Can you work these out from the drawing? Everything is in mm from the part's minimum corner. A direction names the side the tool comes from. Round coordinates to 2 decimals unless told otherwise and drop trailing zeros. Order: outer loops, then holes, each group sorted by start corner. A loop starts at its lowest first (then second) coordinate and runs counter-clockwise, first axis right, second up. Notation, with made-up numbers: (-16.75, -2.75) - (-0.75, -2.75) arc R24 cw to (-0.75, 7.25) - close; hole circle Ø8 at (62.25, 49). An arc over 180 degrees is marked (long way). Answer as a JSON object with one key per item and string values.
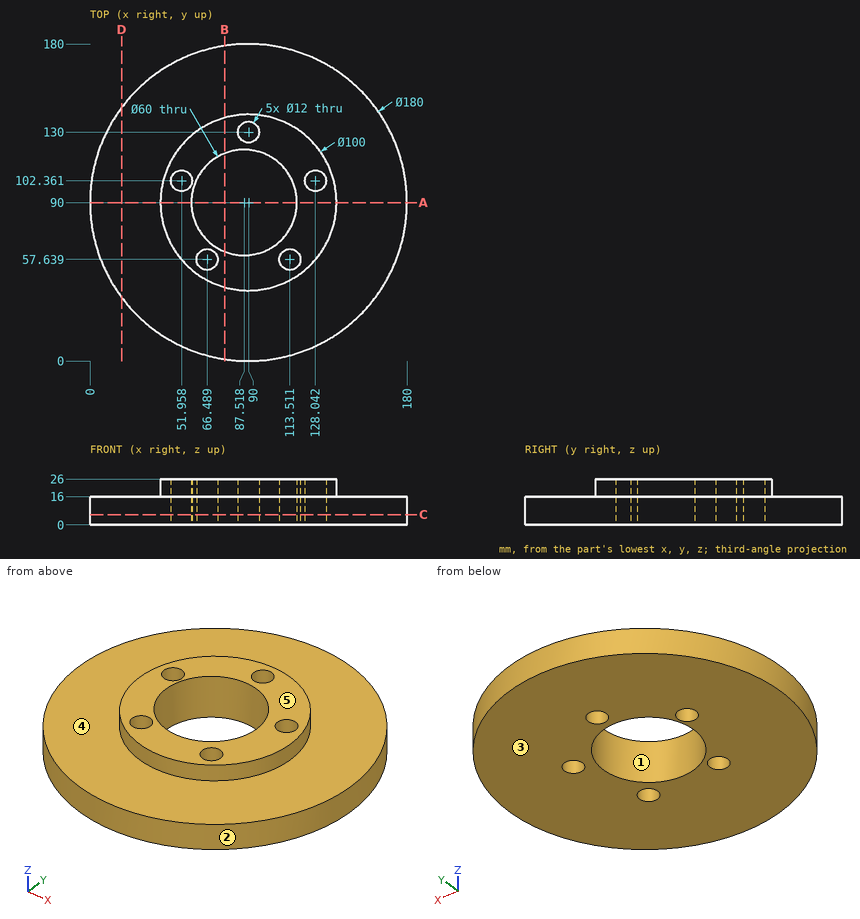
1. Imagine slicing it at C-C (z = 5.75). List the corners of the cut face in (x, y) for me, plus the area to 3 significant figures.
Responses:
{"outline": "circle Ø180 at (90, 90); hole circle Ø12 at (51.96, 102.36); hole circle Ø60 at (87.52, 90); hole circle Ø12 at (66.49, 57.64); hole circle Ø12 at (90, 130); hole circle Ø12 at (113.51, 57.64); hole circle Ø12 at (128.04, 102.36)", "area": "22,100 mm2"}
2. If I drill on L1, parallel to Y at x = 94.5, z = 12.75 (1 decimal); L2, parallel to Y at x = 114, z = 11.5 (1 decimal); L3, parallel to Z at x = 44.5, y = 50, over which ranges is the centre line in solid material (lowest first)? Write a range as [from, to].
Responses:
{"L1": "[0.1, 60.8], [119.2, 126], [134, 179.9]", "L2": "[3.3, 51.7], [63.6, 75.9], [104.1, 176.7]", "L3": "[0, 16]"}
3. Imagine slicing it at D-D (x = 18). List the corners of the cut face in (y, z) for me.
Responses:
{"outline": "(36, 0) - (144, 0) - (144, 16) - (36, 16) - close"}
4. Imagine slicing it at A-A (y = 90). List the corners of the cut face in (x, z) for me.
Responses:
{"outline": "(0, 0) - (57.52, 0) - (57.52, 26) - (40, 26) - (40, 16) - (0, 16) - close; (117.52, 0) - (180, 0) - (180, 16) - (140, 16) - (140, 26) - (117.52, 26) - close"}
5. For the marked faces 4 and 5, which set-ups out of +Z, -Z, +X, -X, +Y, -Y let a thin tool reach every point of the face, with its end or its side?
Responses:
{"face 4": "+Z", "face 5": "+Z, +X, -X, +Y, -Y"}
6. Thinking about a two-plate mould opening in X: for the marked faces 1, 2 and 3, which applies, pulls with the +X half, pulls with the -X half, needs draft (parallel to the pull), parting line crosses it, or undercut?
Responses:
{"face 1": "undercut", "face 2": "parting line crosses it", "face 3": "needs draft"}
7. For P1, Ø12, axis at x = 102, z = 19, coming from the +Y side; P2, Ø2, axis at y = 44.5, z = 14, coming from the +X side; P3, Ø6, axis at x = 105, z = 20, coming from the -Y side; P4, Ø11, axis at x = 66.49, y = 57.64, coming from the +Z side, each with a flat end and sliding along its axis, tell me the tip position at first contact or that it passes through.
Responses:
{"P1": "y = 179.74", "P2": "x = 168.23", "P3": "y = 41.46", "P4": "through"}
8. Imagine slicing it at B-B (x = 76.5). List the corners of the cut face in (y, z) for me, plus the area to 3 significant figures.
Responses:
{"outline": "(1.02, 0) - (62.1, 0) - (62.1, 26) - (41.86, 26) - (41.86, 16) - (1.02, 16) - close; (117.9, 0) - (178.98, 0) - (178.98, 16) - (138.14, 16) - (138.14, 26) - (117.9, 26) - close", "area": "2,360 mm2"}
